```python
from build123d import *

# Parameters (mm, degrees)
MODEL_R                 = 8.05
MODEL_R_2               = 1
MODEL_W                 = 25.8
MODEL_H                 = 11.3
MODEL_W_2               = 11.8
MODEL_H_2               = 22.5
SALIENTE_EXTRUIR1_DEPTH = 3
CROQUIS2_W              = 38.3
CROQUIS2_H              = 12.1
CORTAR_EXTRUIR1_DEPTH   = 1
CROQUIS3_R              = 1.5
CORTAR_EXTRUIR2_DEPTH   = 1
CROQUIS4_W              = 20
CROQUIS4_H              = 3
SALIENTE_EXTRUIR2_DEPTH = 8
CROQUIS5_R              = 1.5
CORTAR_EXTRUIR3_DEPTH   = 3
CROQUIS6_R              = 2.25
CORTAR_EXTRUIR4_DEPTH   = 1
REDONDEO1_R             = 2


with BuildPart() as part:
    # Model → Saliente-Extruir1 (new body)
    with BuildSketch(Plane.XY):
        with BuildLine():
            Line((50.589823504, -56.021207572), (70.589823504, -56.021207572))
            Line((70.589823504, -56.021207572), (70.589823504, -55.020997464))
            ThreePointArc((70.589823504, -55.020997464), (71.175609941, -53.606783901), (72.589823504, -53.020997464))
            Line((72.589823504, -53.020997464), (88.870799912, -53.020997464))
            Line((88.870799912, -53.020997464), (109.670799912, -53.020997464))
            ThreePointArc((109.670799912, -53.020997464), (111.085013474, -52.435211026), (111.670799912, -51.020997464))
            Line((111.670799912, -51.020997464), (111.670799912, -21.120997464))
            ThreePointArc((111.670799912, -21.120997464), (111.085013474, -19.706783901), (109.670799912, -19.120997464))
            Line((109.670799912, -19.120997464), (92.870799912, -19.120997464))
            ThreePointArc((92.870799912, -19.120997464), (91.456586349, -18.535211026), (90.870799912, -17.120997464))
            Line((90.870799912, -17.120997464), (90.870799912, 1.979002536))
            ThreePointArc((90.870799912, 1.979002536), (90.150187884, 3.212884764), (88.940527152, 3.973455574))
            ThreePointArc((88.940527152, 3.973455574), (82.556801864, 7.967186508), (80.592387516, 15.236499516))
            ThreePointArc((80.592387516, 15.236499516), (73.016137183, 12.831206377), (66.424253692, 8.389126209))
            ThreePointArc((66.424253692, 8.389126209), (62.464845981, 11.66270114), (60.387431279, 16.361376528))
            ThreePointArc((60.387431279, 16.361376528), (55.039384462, 14.426569266), (50.461877073, 11.051438157))
            ThreePointArc((50.461877073, 11.051438157), (49.41482724, 13.546636971), (50.438823204, 16.051385009))
            ThreePointArc((50.438823204, 16.051385009), (43.800023098, 13.634815248), (38.471226177, 8.99613013))
            ThreePointArc((38.471226177, 8.99613013), (37.976525569, 11.673196605), (38.618250464, 14.318872844))
            ThreePointArc((38.618250464, 14.318872844), (33.077419178, 10.94136051), (30.527119253, 4.974420659))
            Line((30.527119253, 4.974420659), (30.527119253, -17.120997464))
            ThreePointArc((30.527119253, -17.120997464), (29.941332816, -18.535211026), (28.527119253, -19.120997464))
            Line((28.527119253, -19.120997464), (11.727119253, -19.120997464))
            ThreePointArc((11.727119253, -19.120997464), (10.312905691, -19.706783901), (9.727119253, -21.120997464))
            Line((9.727119253, -21.120997464), (9.727119253, -51.076893199))
            ThreePointArc((9.727119253, -51.076893199), (10.296410138, -52.451282972), (11.670799912, -53.020573857))
            Line((11.670799912, -53.020573857), (32.527119253, -53.020997464))
            Line((32.527119253, -53.020997464), (48.589823504, -53.020997464))
            ThreePointArc((48.589823504, -53.020997464), (50.004037066, -53.606783901), (50.589823504, -55.020997464))
            Line((50.589823504, -55.020997464), (50.589823504, -56.021207572))
        make_face()
        with Locations((47.589823504, -8.020840193)):
            Circle(MODEL_R, mode=Mode.SUBTRACT)
        with Locations((73.589823504, -8.020840193)):
            Circle(MODEL_R, mode=Mode.SUBTRACT)
        with Locations((102.770799912, -21.720997464)):
            Circle(MODEL_R_2, mode=Mode.SUBTRACT)
        with Locations((102.770799912, -49.020997464)):
            Circle(MODEL_R_2, mode=Mode.SUBTRACT)
        with Locations((18.627119253, -21.720997464)):
            Circle(MODEL_R_2, mode=Mode.SUBTRACT)
        with Locations((18.627119253, -49.020997464)):
            Circle(MODEL_R_2, mode=Mode.SUBTRACT)
        with Locations((60.589823504, -33.326919867)):
            Rectangle(MODEL_W, MODEL_H, mode=Mode.SUBTRACT)
        with Locations((102.770799912, -35.370997464)):
            Rectangle(MODEL_W_2, MODEL_H_2, mode=Mode.SUBTRACT)
        with Locations((18.627119253, -35.370997464)):
            Rectangle(MODEL_W_2, MODEL_H_2, mode=Mode.SUBTRACT)
    extrude(amount=SALIENTE_EXTRUIR1_DEPTH)

    # Croquis2 → Cortar-Extruir1 (cut)
    with BuildSketch(Plane(origin=(0, 0, 0), x_dir=(-1, 0, 0), z_dir=(0, 0, -1))):
        with Locations((-61.789823504, -33.326919867)):
            Rectangle(CROQUIS2_W, CROQUIS2_H)
    extrude(amount=-CORTAR_EXTRUIR1_DEPTH, mode=Mode.SUBTRACT)

    # Croquis3 → Cortar-Extruir2 (cut)
    with BuildSketch(Plane.XY.offset(3)):
        with Locations((18.627119253, -21.720997464)):
            Circle(CROQUIS3_R)
        with Locations((18.627119253, -49.020997464)):
            Circle(CROQUIS3_R)
        with Locations((102.770799912, -49.020997464)):
            Circle(CROQUIS3_R)
        with Locations((102.770799912, -21.720997464)):
            Circle(CROQUIS3_R)
    extrude(amount=-CORTAR_EXTRUIR2_DEPTH, mode=Mode.SUBTRACT)

    # Croquis4 → Saliente-Extruir2 (add)
    with BuildSketch(Plane(origin=(0, 0, 0), x_dir=(-1, 0, 0), z_dir=(0, 0, -1))):
        with Locations((-60.589823504, -54.521207572)):
            Rectangle(CROQUIS4_W, CROQUIS4_H)
    extrude(amount=SALIENTE_EXTRUIR2_DEPTH)

    # Croquis5 → Cortar-Extruir3 (cut)
    with BuildSketch(Plane(origin=(0, -53.021207572, 0), x_dir=(1, 0, 0), z_dir=(0, 1, 0))):
        with Locations((54.589823504, 3.5)):
            Circle(CROQUIS5_R)
        with Locations((66.589823504, 3.5)):
            Circle(CROQUIS5_R)
    extrude(amount=-CORTAR_EXTRUIR3_DEPTH, mode=Mode.SUBTRACT)

    # Croquis6 → Cortar-Extruir4 (cut)
    with BuildSketch(Plane(origin=(0, -53.021207572, 0), x_dir=(1, 0, 0), z_dir=(0, 1, 0))):
        with Locations((66.589823504, 3.5)):
            Circle(CROQUIS6_R)
        with Locations((54.589823504, 3.5)):
            Circle(CROQUIS6_R)
    extrude(amount=-CORTAR_EXTRUIR4_DEPTH, mode=Mode.SUBTRACT)

    # Redondeo1
    redondeo1_edges = [part.edges().sort_by_distance(p)[0] for p in [
        (70.589823504, -54.521207572, -8),
        (50.589823504, -54.521207572, -8),
    ]]
    fillet(redondeo1_edges, radius=REDONDEO1_R)


solid = part.part
```
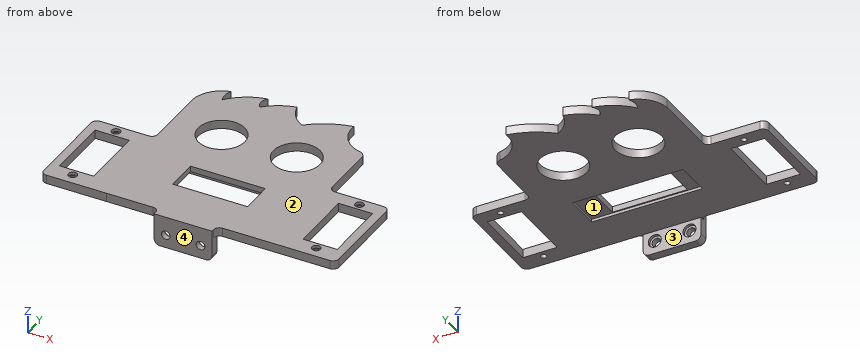
Build history of the part. All positions in model axes, mm. Face numbers are marked on the shaded views. A direction names the side the tool comes from. Round coordinates to 2 decimals unless told otherwise and drop trailing zeros. Order: outer loops, then holes, each group sorted by start corner. A loop starts at its lowest first (then second) coordinate and runs counter-clockwise, first axis right, second up. Notation, with made-up numbers: (-40, 79.5) -> (-23, 79.5) arc R24 ccw to (-23, 89.5) -> close; hole circle Ø8 at (71.5, 34). An arc over 180 degrees is marked (long way). Answer in a Markdown table with one row per item.
1) Band-saw the part on A-A on y = -35. Give the cut face in (x, z).
Values:
| item | result |
|---|---|
| outline | (9.73, 0) -> (12.73, 0) -> (12.73, 3) -> (9.73, 3) -> close; (24.53, 0) -> (42.64, 0) -> (42.64, 1) -> (47.69, 1) -> (47.69, 3) -> (24.53, 3) -> close; (73.49, 1) -> (80.94, 1) -> (80.94, 0) -> (96.87, 0) -> (96.87, 3) -> (73.49, 3) -> close; (108.67, 0) -> (111.67, 0) -> (111.67, 3) -> (108.67, 3) -> close |
2) Pin check, flat tips, straight feed: P1, Ø5, axis at x = 23.5, y = -45, coming from the -Z side; P2, Ø3.5, axis at x = 93.5, z = 1.5, coming from the -Y side; P3, Ø2, axis at x = 54.5, z = -4.5, coming from the +Y side; P4, Ø1.5, axis at x = 18.5, y = -49, coming from the +Z side. Stop position of each tip, or through.
Values:
| item | result |
|---|---|
| P1 | z = 0 |
| P2 | y = -53.02 |
| P3 | y = -54.02 |
| P4 | through |
3) Mould opens along X. For the marked faces 1 and 2 say: released by +X, released by -X, zero draft, split by the parting line, or undercut.
Values:
| item | result |
|---|---|
| face 1 | undercut |
| face 2 | zero draft |
4) Band-saw the part on B-B on z = -3.5. Give the cut face in (x, y).
Values:
| item | result |
|---|---|
| outline | (50.59, -56.02) -> (53.09, -56.02) -> (53.09, -54.02) -> (52.34, -54.02) -> (52.34, -53.02) -> (50.59, -53.02) -> close; (56.09, -56.02) -> (65.09, -56.02) -> (65.09, -54.02) -> (64.34, -54.02) -> (64.34, -53.02) -> (56.84, -53.02) -> (56.84, -54.02) -> (56.09, -54.02) -> close; (68.09, -56.02) -> (70.59, -56.02) -> (70.59, -53.02) -> (68.84, -53.02) -> (68.84, -54.02) -> (68.09, -54.02) -> close |
5) Which spindle directions (+Z, -Z, +X, -X, +Y, -Y) get a long thin tool onto all of the face, cutting with end or side? Do the marked faces 3 and 4. Say none if no direction does.
Values:
| item | result |
|---|---|
| face 3 | -Z, +X, -X, +Y |
| face 4 | +Z, -Z, +X, -X, -Y |
6) Band-saw the part on D-D on x = 84. Give the cut face in (y, z), and give its area (3 significant figures).
Values:
| item | result |
|---|---|
| outline | (-53.02, 0) -> (6.39, 0) -> (6.39, 3) -> (-53.02, 3) -> close |
| area | 178 mm2 |
7) Band-saw the part on C-C on y = 7. Give the cut face in (x, z).
Values:
| item | result |
|---|---|
| outline | (30.92, 0) -> (83.37, 0) -> (83.37, 3) -> (30.92, 3) -> close |
8) Wall check: L1, parallel to X at y = -55.6, z = -3.5; L2, parallel to Y at x = 97.5, z = 2.5; L3, parallel to X at y = -53.65, z = -3.5. Give the ranges that are in metal, low to high.
Values:
| item | result |
|---|---|
| L1 | 50.59 to 53.09, 56.09 to 65.09, 68.09 to 70.59 |
| L2 | -53.02 to -46.62, -24.12 to -19.12 |
| L3 | 50.59 to 52.34, 56.84 to 64.34, 68.84 to 70.59 |
